Design review of the part built by this model. Coordinates are the model's own, in mm. Coordinates: 2 decimals unless noted, no trailing zeros. Loops run counter-clockwise (first coordinate to the right, second up) from the corner with the lowest first, then second, coordinate; pieces in that order, holes last. Notation, with made-up numbers: (23, 29.5) -> (74, 29.5) arc R27 cw to (74, 46.5) -> close; hole circle Ø10 at (71, -15). An arc over 180 degrees is marked (long way). Answer as a JSON object with one key per item and string values.
```python
from build123d import *

# Parameters (mm, degrees)
F0_R     = 241.3
F1_DEPTH = 25.4


with BuildPart() as f1:
    # F0 (on Top) → F1 (new body)
    with BuildSketch(Plane.XY):
        with BuildLine():
            ThreePointArc((-80.9625, -140.231164), (80.9625, -140.231164), (161.925, 0))
            ThreePointArc((161.925, 0), (-80.9625, 140.231164), (-80.9625, -140.231164))
        make_face()
        Circle(F0_R)
        with BuildLine():
            ThreePointArc((-95.860263, -193.451854), (-114.807712, -198.852791), (-119.604089, -179.74335))
            ThreePointArc((-119.604089, -179.74335), (-152.664354, -152.664354), (-179.74335, -119.604089))
            ThreePointArc((-179.74335, -119.604089), (-198.852791, -114.807712), (-193.451854, -95.860263))
            ThreePointArc((-193.451854, -95.860263), (-208.543386, -55.879032), (-215.464352, -13.708504))
            ThreePointArc((-215.464352, -13.708504), (-229.615425, 0), (-215.464352, 13.708504))
            ThreePointArc((-215.464352, 13.708504), (-208.543386, 55.879032), (-193.451854, 95.860263))
            ThreePointArc((-193.451854, 95.860263), (-198.852791, 114.807712), (-179.74335, 119.604089))
            ThreePointArc((-179.74335, 119.604089), (-152.664354, 152.664354), (-119.604089, 179.74335))
            ThreePointArc((-119.604089, 179.74335), (-114.807712, 198.852791), (-95.860263, 193.451854))
            ThreePointArc((-95.860263, 193.451854), (-55.879032, 208.543386), (-13.708504, 215.464352))
            ThreePointArc((-13.708504, 215.464352), (-0.217852, 229.613695), (13.715425, 215.9))
            ThreePointArc((13.715425, 215.9), (13.713695, 215.682148), (13.708504, 215.464352))
            ThreePointArc((13.708504, 215.464352), (55.879032, 208.543386), (95.860263, 193.451854))
            ThreePointArc((95.860263, 193.451854), (111.288937, 200.277681), (121.665425, 186.974885))
            ThreePointArc((121.665425, 186.974885), (121.140028, 183.215091), (119.604089, 179.74335))
            ThreePointArc((119.604089, 179.74335), (152.664354, 152.664354), (179.74335, 119.604089))
            ThreePointArc((179.74335, 119.604089), (193.643067, 119.935334), (200.69031, 107.95))
            ThreePointArc((200.69031, 107.95), (198.742367, 100.904488), (193.451854, 95.860263))
            ThreePointArc((193.451854, 95.860263), (208.543386, 55.879032), (215.464352, 13.708504))
            ThreePointArc((215.464352, 13.708504), (225.443002, 9.851091), (229.615425, 0))
            ThreePointArc((229.615425, 0), (225.443002, -9.851091), (215.464352, -13.708504))
            ThreePointArc((215.464352, -13.708504), (208.543386, -55.879032), (193.451854, -95.860263))
            ThreePointArc((193.451854, -95.860263), (198.742367, -100.904488), (200.69031, -107.95))
            ThreePointArc((200.69031, -107.95), (193.643067, -119.935334), (179.74335, -119.604089))
            ThreePointArc((179.74335, -119.604089), (152.664354, -152.664354), (119.604089, -179.74335))
            ThreePointArc((119.604089, -179.74335), (121.140028, -183.215091), (121.665425, -186.974885))
            ThreePointArc((121.665425, -186.974885), (111.288937, -200.277681), (95.860263, -193.451854))
            ThreePointArc((95.860263, -193.451854), (55.879032, -208.543386), (13.708504, -215.464352))
            ThreePointArc((13.708504, -215.464352), (13.713695, -215.682148), (13.715425, -215.9))
            ThreePointArc((13.715425, -215.9), (-0.217852, -229.613695), (-13.708504, -215.464352))
            ThreePointArc((-13.708504, -215.464352), (-55.879032, -208.543386), (-95.860263, -193.451854))
        make_face(mode=Mode.SUBTRACT)
        with BuildLine():
            ThreePointArc((-119.604089, -179.74335), (-111.288937, -173.672089), (-101.092288, -175.096978))
            ThreePointArc((-101.092288, -175.096978), (-96.072094, -180.117172), (-94.234575, -186.974885))
            ThreePointArc((-94.234575, -186.974885), (-94.647204, -190.313822), (-95.860263, -193.451854))
            ThreePointArc((-95.860263, -193.451854), (-55.879032, -208.543386), (-13.708504, -215.464352))
            ThreePointArc((-13.708504, -215.464352), (0, -202.184575), (13.708504, -215.464352))
            ThreePointArc((13.708504, -215.464352), (55.879032, -208.543386), (95.860263, -193.451854))
            ThreePointArc((95.860263, -193.451854), (101.092288, -175.096978), (119.604089, -179.74335))
            ThreePointArc((119.604089, -179.74335), (152.664354, -152.664354), (179.74335, -119.604089))
            ThreePointArc((179.74335, -119.604089), (175.096978, -101.092288), (193.451854, -95.860263))
            ThreePointArc((193.451854, -95.860263), (208.543386, -55.879032), (215.464352, -13.708504))
            ThreePointArc((215.464352, -13.708504), (202.184575, 0), (215.464352, 13.708504))
            ThreePointArc((215.464352, 13.708504), (208.543386, 55.879032), (193.451854, 95.860263))
            ThreePointArc((193.451854, 95.860263), (175.096978, 101.092288), (179.74335, 119.604089))
            ThreePointArc((179.74335, 119.604089), (152.664354, 152.664354), (119.604089, 179.74335))
            ThreePointArc((119.604089, 179.74335), (101.092288, 175.096978), (95.860263, 193.451854))
            ThreePointArc((95.860263, 193.451854), (55.879032, 208.543386), (13.708504, 215.464352))
            ThreePointArc((13.708504, 215.464352), (0, 202.184575), (-13.708504, 215.464352))
            ThreePointArc((-13.708504, 215.464352), (-55.879032, 208.543386), (-95.860263, 193.451854))
            ThreePointArc((-95.860263, 193.451854), (-94.647204, 190.313822), (-94.234575, 186.974885))
            ThreePointArc((-94.234575, 186.974885), (-104.190206, 173.784857), (-119.604089, 179.74335))
            ThreePointArc((-119.604089, 179.74335), (-152.664354, 152.664354), (-179.74335, 119.604089))
            ThreePointArc((-179.74335, 119.604089), (-174.989551, 114.618182), (-173.25946, 107.95))
            ThreePointArc((-173.25946, 107.95), (-179.929372, 96.182518), (-193.451854, 95.860263))
            ThreePointArc((-193.451854, 95.860263), (-208.543386, 55.879032), (-215.464352, 13.708504))
            ThreePointArc((-215.464352, 13.708504), (-206.048909, 9.543002), (-202.184575, 0))
            ThreePointArc((-202.184575, 0), (-206.048909, -9.543002), (-215.464352, -13.708504))
            ThreePointArc((-215.464352, -13.708504), (-208.543386, -55.879032), (-193.451854, -95.860263))
            ThreePointArc((-193.451854, -95.860263), (-179.929372, -96.182518), (-173.25946, -107.95))
            ThreePointArc((-173.25946, -107.95), (-174.989551, -114.618182), (-179.74335, -119.604089))
            ThreePointArc((-179.74335, -119.604089), (-152.664354, -152.664354), (-119.604089, -179.74335))
        make_face()
        with BuildLine():
            ThreePointArc((-80.9625, -140.231164), (-80.9625, 140.231164), (161.925, 0))
            ThreePointArc((161.925, 0), (80.9625, -140.231164), (-80.9625, -140.231164))
        make_face(mode=Mode.SUBTRACT)
    extrude(amount=F1_DEPTH)


solid = f1.part
```
1) Add section D-D, the plane z = 5. Count the separate pieces of the cut face and the enclosed holes in it, and give its area (3 significant figures).
Completed:
{"separate pieces": "1", "enclosed holes": "13", "area": "93,500 mm²"}
2) Add section C-C, the plane x = 149.5. Give the boundary of the cut face in (y, z).
Completed:
{"outline": "(-189.41, 0) -> (-62.2, 0) -> (-62.2, 25.4) -> (-189.41, 25.4) -> close; (62.2, 0) -> (189.41, 0) -> (189.41, 25.4) -> (62.2, 25.4) -> close"}
3) Wall thickness on probe 1 along Y at (x, z) = (0, 12.75) (3 decimals); probe 2 along X at (y, z) = (194, 14); probe 3 along X at (y, z) = (117, 23.5): over which ranges is each line inside the solid? List them lowest first.
Completed:
{"probe 1": "-241.3 to -229.615, -202.185 to -161.925, 161.925 to 202.185, 229.615 to 241.3", "probe 2": "-143.49 to -119.73, -96.17 to 96.17, 119.73 to 143.49", "probe 3": "-211.04 to -197.28, -176.67 to -111.94, 111.94 to 176.67, 197.28 to 211.04"}
4) Add section A-A, the plane y = 39.5. Give the boundary of the cut face in (x, z).
Completed:
{"outline": "(-238.05, 0) -> (-157.03, 0) -> (-157.03, 25.4) -> (-238.05, 25.4) -> close; (157.03, 0) -> (238.05, 0) -> (238.05, 25.4) -> (157.03, 25.4) -> close"}
5) Clearance check with flat-ended pins moving along their axes: pin 1 Ø1 at (y, z) = (77, 18) entering from +X; pin 2 Ø8 at (x, z) = (-171.5, 4) entering from -Y; pin 3 Ø4 at (x, z) = (-103.5, 19.5) entering from +Y. State where each tip first meets the part, or that it passes through.
Completed:
{"pin 1": "x = 228.85", "pin 2": "y = -173.69", "pin 3": "y = 218.91"}
6) Add section B-B, the plane x = 0. Give the boundary of the cut face in (y, z) (3 decimals), and give its area (3 significant figures).
Completed:
{"outline": "(-241.3, 0) -> (-229.615, 0) -> (-229.615, 25.4) -> (-241.3, 25.4) -> close; (-202.185, 0) -> (-161.925, 0) -> (-161.925, 25.4) -> (-202.185, 25.4) -> close; (161.925, 0) -> (202.185, 0) -> (202.185, 25.4) -> (161.925, 25.4) -> close; (229.615, 0) -> (241.3, 0) -> (241.3, 25.4) -> (229.615, 25.4) -> close", "area": "2,640 mm²"}
